```python
from build123d import *

# Parameters (mm, degrees)
SKETCH_2_R          = 1.5
CUT_EXTRUDE_1_DEPTH = 34.88583775
SKETCH_4_R          = 14
SKETCH_4_R_2        = 12.75
CUT_EXTRUDE_4_DEPTH = 34.88583775
CUT_EXTRUDE_5_DEPTH = 3
SKETCH_6_R          = 4
CUT_EXTRUDE_6_DEPTH = 47.627513337


with BuildPart() as part:
    # 草图1 → 旋转1 (revolve)
    with BuildSketch(Plane(origin=(0, 0, 0), x_dir=(0, 0, -1), z_dir=(1, 0, 0)), mode=Mode.PRIVATE) as revolve_1_sk:
        Polygon((-21.5, 0), (-21.5, 6), (-13.5, 6), (-13.5, 7), (-6, 7), (-6, 14), (6, 14), (6, 7), (13.5, 7), (13.5, 6), (21.5, 6), (21.5, 0), align=None)
    revolve(revolve_1_sk.sketch.rotate(Axis((0, 0, 21.5), (0, 0, -1)), 90), axis=Axis((0, 0, 21.5), (0, 0, -1)))

    # 草图2 → 切除-拉伸1 (cut, through all)
    with BuildSketch(Plane.XY.offset(6)):
        with Locations((0, 10.5)):
            Circle(SKETCH_2_R)
        with Locations((10.5, 0)):
            Circle(SKETCH_2_R)
        with Locations((0, -10.5)):
            Circle(SKETCH_2_R)
        with Locations((-10.5, 0)):
            Circle(SKETCH_2_R)
    extrude(amount=-CUT_EXTRUDE_1_DEPTH, mode=Mode.SUBTRACT)

    # 草图4 → 切除-拉伸4 (cut, through all)
    with BuildSketch(Plane(origin=(0, 0, -6), x_dir=(-1, 0, 0), z_dir=(0, 0, -1))):
        Circle(SKETCH_4_R)
        Circle(SKETCH_4_R_2, mode=Mode.SUBTRACT)
    extrude(amount=-CUT_EXTRUDE_4_DEPTH, mode=Mode.SUBTRACT)

    # 草图5 → 切除-拉伸5 (cut)
    with BuildSketch(Plane(origin=(0, 0, -6), x_dir=(-1, 0, 0), z_dir=(0, 0, -1))):
        with BuildLine():
            Line((-11.313708499, 4), (-8.485281374, 3))
            ThreePointArc((-8.485281374, 3), (-6.363961031, 6.363961031), (-3, 8.485281374))
            Line((-3, 8.485281374), (-4, 11.313708499))
            ThreePointArc((-4, 11.313708499), (-8.485281374, 8.485281374), (-11.313708499, 4))
        make_face()
        with BuildLine():
            Line((4, 11.313708499), (3, 8.485281374))
            ThreePointArc((3, 8.485281374), (6.363961031, 6.363961031), (8.485281374, 3))
            Line((8.485281374, 3), (11.313708499, 4))
            ThreePointArc((11.313708499, 4), (8.485281374, 8.485281374), (4, 11.313708499))
        make_face()
        with BuildLine():
            Line((11.313708499, -4), (8.485281374, -3))
            ThreePointArc((8.485281374, -3), (6.363961031, -6.363961031), (3, -8.485281374))
            Line((3, -8.485281374), (4, -11.313708499))
            ThreePointArc((4, -11.313708499), (8.485281374, -8.485281374), (11.313708499, -4))
        make_face()
        with BuildLine():
            Line((-4, -11.313708499), (-3, -8.485281374))
            ThreePointArc((-3, -8.485281374), (-6.363961031, -6.363961031), (-8.485281374, -3))
            Line((-8.485281374, -3), (-11.313708499, -4))
            ThreePointArc((-11.313708499, -4), (-8.485281374, -8.485281374), (-4, -11.313708499))
        make_face()
    cut_extrude_5 = extrude(amount=-CUT_EXTRUDE_5_DEPTH, mode=Mode.SUBTRACT)

    # 镜向2: 切除-拉伸5 across plane
    add(cut_extrude_5.mirror(Plane.XY), mode=Mode.SUBTRACT)

    # 草图6 → 切除-拉伸6 (cut, through all)
    with BuildSketch(Plane(origin=(0, 0, -21.5), x_dir=(-1, 0, 0), z_dir=(0, 0, -1))):
        Circle(SKETCH_6_R)
    extrude(amount=-CUT_EXTRUDE_6_DEPTH, mode=Mode.SUBTRACT)


solid = part.part
```
Input: part model. Units: mm. Frame: model coordinates. A direction names the side the tool comes from. Give positions to 0.01 mm unless a question says otherwise; leave off trailing zeros. Loops run counter-clockwise (first coordinate to the right, second up) from the corner with the lowest first, then second, coordinate; pieces in that order, holes last.
1) Section query C-C on x = -10.75. Return the cut outline in (y, z), and give its area (3 significant figures).
A:
outline: (-6.86, -6) - (-5.33, -6) - (-5.33, -3) - (-3.8, -3) - (-3.8, -6) - (-1.48, -6) - (-1.48, 6) - (-3.8, 6) - (-3.8, 3) - (-5.33, 3) - (-5.33, 6) - (-6.86, 6) - close; (1.48, -6) - (3.8, -6) - (3.8, -3) - (5.33, -3) - (5.33, -6) - (6.86, -6) - (6.86, 6) - (5.33, 6) - (5.33, 3) - (3.8, 3) - (3.8, 6) - (1.48, 6) - close
area: 111 mm2
2) Reachability of faces 1 (the cylindrical face through (3.23, 6.21, 9.7)), 2 (the cylindrical face through (-12, 0, 0)), 3 (the cylindrical face through (3.23, 6.21, -9.8)) from +Z, -Z, +X, -X, +Y, -Y: full face, straight path, thin tool, end or side. Return the list, or none.
A:
face 1: +Z
face 2: +Z, -Z
face 3: -Z
3) Line query: L1, parallel to Y at x = 0, z = -0.25; L2, parallel to X at y = 5, z = 4.5; L3, parallel to Z at x = 9, y = 8.5. Output: solid intervals per line, ascending.
A:
L1: y = -12.75 to -12, -9 to -4, 4 to 9, 12 to 12.75
L2: x = -11.73 to -10.91, -7.48 to 7.48, 10.91 to 11.73
L3: z = -6 to 6
4) Section query A-A on x = 0. Count the separate pieces of the cut face and the enclosed holes in it, and give its area (3 significant figures).
A:
separate pieces: 4
enclosed holes: 0
area: 292 mm2
5) Contact query for flat-ended pins moving along their axis: pin 1 (12 mm diameter, centred on x = 1, z = -10, fed in from -Y); pin 2 (2.5 mm diameter, centred on x = -6.5, y = -6.5, fed in from +Z); pin 3 (4 mm diameter, centred on x = 6.5, y = -6, fed in from +Z); pin 4 (1.5 mm diameter, centred on y = -2, z = -6, fed in from +X). Output: stop coordinate, or through.
A:
pin 1: stops at y = -12.75
pin 2: stops at z = 6
pin 3: stops at z = 13.5
pin 4: stops at x = 12.69
6) Section query B-B on y = 2.5. Return the cut outline in (x, z).
A:
outline: (-12.5, -6) - (-6.54, -6) - (-6.54, -13.5) - (-5.45, -13.5) - (-5.45, -21.5) - (-3.12, -21.5) - (-3.12, 21.5) - (-5.45, 21.5) - (-5.45, 13.5) - (-6.54, 13.5) - (-6.54, 6) - (-12.5, 6) - close; (3.12, -21.5) - (5.45, -21.5) - (5.45, -13.5) - (6.54, -13.5) - (6.54, -6) - (12.5, -6) - (12.5, 6) - (6.54, 6) - (6.54, 13.5) - (5.45, 13.5) - (5.45, 21.5) - (3.12, 21.5) - close
